Could you check a few things on this model? Use its own coordinates, in mm. Face numbers are marked on the shaded views. Round coordinates to 2 decimals unless told otherwise and drop trailing zeros. Loops run counter-clockwise (first coordinate to the right, second up) from the corner with the lowest first, then second, coordinate; pieces in that order, holes last. Notation, with made-up numbers: M -19.75,78 L -12.75,78 A28 ccw -12.75,102 Z; hole C 79,17 d3. An arc over 180 degrees is marked long. One line per item, written item: value. Start each with the question number.
Q1. I'm going to push a flat-ended pin straight in: pin 1 Ø9 at (x, z) = (40, 10) entering from +Y. Where does the tip first touch, or does it pass through?
Q2. Imagine slicing it at A-A (z = 10). Please give me the cut outline in (x, y).
Q3. Imagine slicing it at B-B (x = 40). Please give me the cut outline in (y, z), then the cut area to 3 significant figures.
Q4. Imagine slicing it at C-C (y = 70.5). Please give me the cut outline in (x, z).
Q5. Thinking about a two-plate mould opening in X: for the marked faces 1, 2, 3 and 4, which applies, released by +X, released by -X, zero draft, split by the parting line, or undercut?
Q6. Please list where these lines run through material, in increasing order: line 1 along Z through (x, y) = (40, 60); line 2 along X through (y, z) = (63.5, 10); line 3 along X through (y, z) = (93, 14.5).
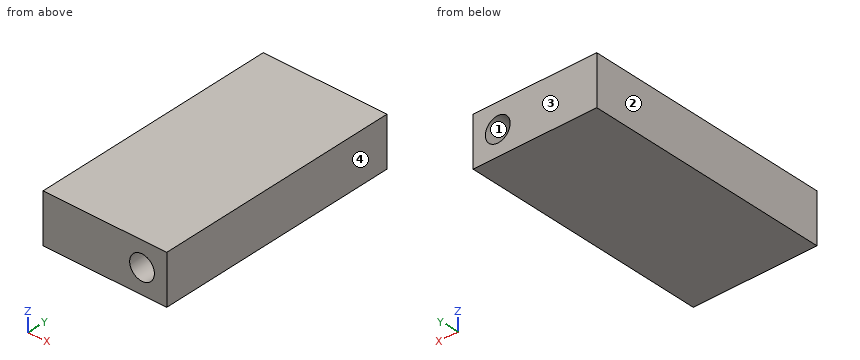
Autodesk Fusion 360 part; units mm, degrees
sketch "Sketch1" plane through (0, 0, 0) normal (0, 1, 0) x (1, 0, 0)
  line L0 (0, 0) -> (50, 0)
  line L1 (50, 0) -> (50, -20)
  line L2 (50, -20) -> (0, -20)
  line L3 (0, -20) -> (0, 0)
  circle A0 centre (40, -10) radius 5
  dimension "d1" = 50
  dimension "d2" = 20
  dimension "d3" = 10
extrude "Extrude1" add sketch "Sketch1" along normal blind 100
Report:
1. pin 1: passes through
2. outline: M 0,0 L 35,0 L 35,100 L 0,100 Z; M 45,0 L 50,0 L 50,100 L 45,100 Z
3. outline: M 0,0 L 100,0 L 100,5 L 0,5 Z; M 0,15 L 100,15 L 100,20 L 0,20 Z
3. area: 1,000 mm²
4. outline: M 0,0 L 50,0 L 50,20 L 0,20 Z; hole C 40,10 d10
5. face 1: undercut
5. face 2: released by -X
5. face 3: zero draft
5. face 4: released by +X
6. line 1: z = 0 to 5, 15 to 20
6. line 2: x = 0 to 35, 45 to 50
6. line 3: x = 0 to 37.82, 42.18 to 50
